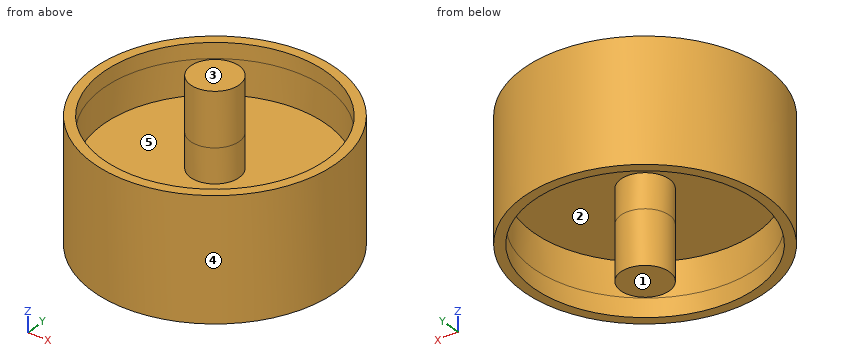
from build123d import *

# Parameters (mm, degrees)
F2_DEPTH = 8.89
F3_DEPTH = 8.89


with BuildPart() as f1:
    # F0 (on Front) → F1 (revolve)
    with BuildSketch(Plane.XZ):
        Polygon((29.21, 15.1165612042), (29.21, 11.1276201193), (29.21, -11.7323798807), (29.21, -16.5423657745), (31.7501313984, -16.5423657745), (31.7501313984, 15.1165612042), align=None)
        Polygon((6.35, 25.0976201193), (0, 25.0976201193), (0, -25.7023798807), (6.35, -25.7023798807), (6.35, -11.7323798807), (29.21, -11.7323798807), (29.21, 11.1276201193), (6.35, 11.1276201193), align=None)
    revolve(axis=Axis((0, 0, -0.3023798807), (0, 0, -1)))

    # F2 (cut): a face of the model
    f2_faces = [f1.faces().sort_by_distance(p)[0] for p in [
        (-28.3838164369, 0, 11.1276201193),
    ]]
    extrude(f2_faces, amount=-F2_DEPTH, mode=Mode.SUBTRACT)

    # F3 (cut): a face of the model
    f3_faces = [f1.faces().sort_by_distance(p)[0] for p in [
        (-7.1761835631, 0, -11.7323798807),
    ]]
    extrude(f3_faces, amount=-F3_DEPTH, mode=Mode.SUBTRACT)


solid = f1.part
Read the model definition and answer for the solid it produces. Units are mm, in the model's axes. Face numbers are marked on the shaded views. A direction names the side the tool comes from. Give positions to 0.01 mm unless a question says otherwise; leave off trailing zeros. Loops run counter-clockwise (first coordinate to the right, second up) from the corner with the lowest first, then second, coordinate; pieces in that order, holes last. Notation, with made-up numbers: M 30,53 L 45,53 A21 cw 45,77 Z; hole C 61.25,8.5 d7. An arc over 180 degrees is marked long. Write each question's results on one line, items separated by ' | '.
1. Straight lines are drawn through the part: line 1 (X direction, y = 0, z = 5); line 2 (Y direction, x = 5, z = -7.5). For each, find the intervals that lie inside material, in ascending order. Write a range as [from, to].
Values:
line 1: x = [-31.75, -29.21], [-6.35, 6.35], [29.21, 31.75] | line 2: y = [-31.35, -28.78], [-3.91, 3.91], [28.78, 31.35]
2. Section C-C on z = -19 is taken. Give the vertices of the cut face in (x, y).
Values:
outline: C 0,0 d12.7
3. Given pin 1 (19 mm diameter, centred on x = 16, y = -10, fed in from -Z); pin 2 (3 mm diameter, centred on y = 14.5, z = 13.5, fed in from -X); pin 3 (12 mm diameter, centred on y = -22, z = -4, fed in from -X); pin 4 (4 mm diameter, centred on y = -20, z = 18.5, fed in from +X), each flat-ended and moving along its own axis, determine where each tip first touches the part or whether it passes through.
Values:
pin 1: stops at z = -2.84 | pin 2: stops at x = -28.97 | pin 3: stops at x = -27.42 | pin 4: passes through
4. The mould has two halves that part along X. Classify the marked faces 3, 4 and 5: pulls with the +X half, pulls with the -X half, needs draft (parallel to the pull), parting line crosses it, or undercut.
Values:
face 3: needs draft | face 4: parting line crosses it | face 5: undercut
5. Section B-B on y = 20 is taken. Give the vertices of the cut face in (x, z).
Values:
outline: M -24.66,-16.54 L -21.29,-16.54 L -21.29,-2.84 L 21.29,-2.84 L 21.29,-16.54 L 24.66,-16.54 L 24.66,15.12 L 21.29,15.12 L 21.29,2.24 L -21.29,2.24 L -21.29,15.12 L -24.66,15.12 Z
6. A tool of negligible diameter and unlimited length cuts with its end or side. For the marked faces 1 and 2, from which of +Z, -Z, +X, -X, +Y, -Y can it reach the whole face along a straight path? Write none if from no direction.
Values:
face 1: -Z, +X, -X, +Y, -Y | face 2: -Z
7. Section A-A on x = 0 is taken. Give the vertices of the cut face in (y, z), plus the area to 3 significant figures.
Values:
outline: M -31.75,-16.54 L -29.21,-16.54 L -29.21,-2.84 L -6.35,-2.84 L -6.35,-25.7 L 6.35,-25.7 L 6.35,-2.84 L 29.21,-2.84 L 29.21,-16.54 L 31.75,-16.54 L 31.75,15.12 L 29.21,15.12 L 29.21,2.24 L 6.35,2.24 L 6.35,25.1 L -6.35,25.1 L -6.35,2.24 L -29.21,2.24 L -29.21,15.12 L -31.75,15.12 Z | area: 1,040 mm^2
8. Section D-D on x = 19.5 is taken. Give the vertices of the cut face in (y, z), plus the area to 3 significant figures.
Values:
outline: M -25.06,-16.54 L -21.75,-16.54 L -21.75,-2.84 L 21.75,-2.84 L 21.75,-16.54 L 25.06,-16.54 L 25.06,15.12 L 21.75,15.12 L 21.75,2.24 L -21.75,2.24 L -21.75,15.12 L -25.06,15.12 Z | area: 430 mm^2
